Input: part model. Units: mm. Frame: model coordinates. Give positions to 0.01 mm unless a question says otherwise; leave off trailing zeros. Order: outer loops, then holes, each group sorted by start corner. A loop starts at its lowest first (then second) coordinate and runs counter-clockwise, first axis right, second up. Notation, with made-up numbers: (30.25, 8) - (79.25, 8) arc R20 cw to (79.25, 23) - close; hole circle Ø8 at (32, -15.75). An arc over 180 degrees is marked (long way). Answer in a Markdown table with one row per item. Add a question column.
1. Section query B-B on x = 8. Return loops of the section in (y, z), and give its area (3 significant figures).
2. Contact query for flat-ended pins moving along their axis: pin 1 (1.5 mm diameter, centred on x = 10.5, z = -262, fed in from -Y); pin 2 (4 mm diameter, centred on x = 7, z = -281.5, fed in from +Y); pin 3 (3 mm diameter, centred on x = 8.5, z = -317, fed in from -Y). Output: stop coordinate, or through.
3. Ray query, line 1 (Y direction, x = 3.5, z = -97.5); line 2 (Z direction, x = 8.25, y = 32); line 3 (X direction, y = 93, z = -298). Return the intervals inside material, ascending. Write a range as [from, to].
```python
from build123d import *

# Parameters (mm, degrees)
BOSS_EXTRUDE1_DEPTH = 12
CHAMFER1_SIZE       = 12


with BuildPart() as part:
    # Sketch1 → Boss-Extrude1 (new body)
    with BuildSketch(Plane(origin=(0, 0, 0), x_dir=(0, 0, -1), z_dir=(1, 0, 0))):
        with BuildLine():
            Line((0, 0), (0, -10))
            Line((0, -10), (40, -10))
            ThreePointArc((40, -10), (48.819660113, -2.639320225), (60, 0))
            Line((60, 0), (315, 0))
            ThreePointArc((315, 0), (326.180339887, -2.639320225), (335, -10))
            Line((335, -10), (375, -10))
            Line((375, -10), (375, 0))
            Line((375, 0), (375, 100))
            Line((375, 100), (0, 100))
            Line((0, 100), (0, 0))
        make_face()
    extrude(amount=BOSS_EXTRUDE1_DEPTH)

    # Chamfer1
    chamfer1_edges = [part.edges().sort_by_distance(p)[0] for p in [
        (0, 45, -375),
        (0, 45, 0),
        (0, 100, -187.5),
    ]]
    chamfer(chamfer1_edges, length=CHAMFER1_SIZE - 0.0001)  # a hair under: the kernel refuses the full size


solid = part.part
```
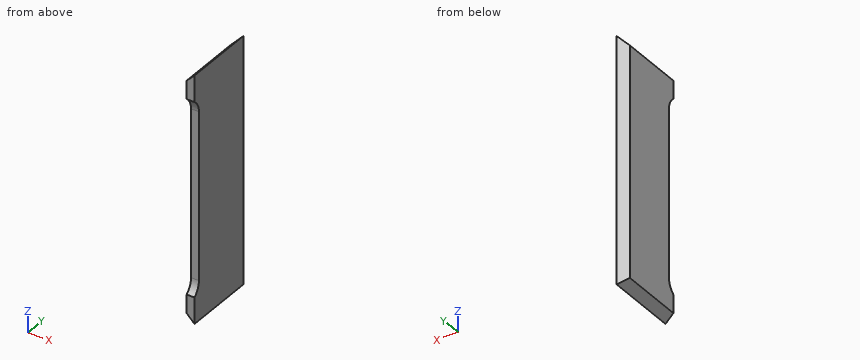
Answer:
| question | item | result |
|---|---|---|
| 1 | outline | (-10, -371) - (96, -371) - (96, -4) - (-10, -4) - (-10, -40) arc R25 cw to (0, -60) - (0, -315) arc R25 cw to (-10, -335) - close |
| 1 | area | 36,100 mm² |
| 2 | pin 1 | stops at y = 0 |
| 2 | pin 2 | stops at y = 97 |
| 2 | pin 3 | stops at y = -0.25 |
| 3 | line 1 | y = [0, 91.5] |
| 3 | line 2 | z = [-371.25, -3.75] |
| 3 | line 3 | x = [5, 12] |
